```python
from build123d import *

# Parameters (mm, degrees)
F0_W      = 18.034
F0_H      = 23.4315
F1_DEPTH  = 21.0566
F2_W      = 18.034
F2_H      = 11.1252
F3_DEPTH  = 13.1699
F4_W      = 12.065
F4_H      = 4.5339
F5_DEPTH  = 12.065
F6_W      = 14.9352
F6_H      = 7.9248
F7_DEPTH  = 11.43
F8_W      = 11.3792
F8_H      = 3.8862
F9_DEPTH  = 11.43
F10_W     = 10.67195
F10_H     = 2.202249
F11_DEPTH = 11.176
F12_W     = 13.372126
F12_H     = 1.887192
F13_DEPTH = 10.922


with BuildPart() as f1:
    # F0 (on Front) → F1 (new body)
    with BuildSketch(Plane.XZ):
        Rectangle(F0_W, F0_H)
    extrude(amount=F1_DEPTH)

    # F2 (on face) → F3 (cut)
    with BuildSketch(Plane.XY.offset(11.71575)):
        with Locations((0, -15.494)):
            Rectangle(F2_W, F2_H)
    extrude(amount=-F3_DEPTH, mode=Mode.SUBTRACT)

    # F4 (on face) → F5 (join)
    with BuildSketch(Plane.XY.offset(11.71575)):
        with Locations((0, -4.9657)):
            Rectangle(F4_W, F4_H)
    extrude(amount=F5_DEPTH)

    # F6 (on face) → F7 (cut)
    with BuildSketch(Plane.XZ.offset(21.0566)):
        with Locations((0, -6.58495)):
            Rectangle(F6_W, F6_H)
    extrude(amount=-F7_DEPTH, mode=Mode.SUBTRACT)

    # F8 (on face) → F9 (cut)
    with BuildSketch(Plane.XY.offset(23.78075)):
        with Locations((0, -4.9657)):
            Rectangle(F8_W, F8_H)
    extrude(amount=-F9_DEPTH, mode=Mode.SUBTRACT)

    # F10 (on face) → F11 (join)
    with BuildSketch(Plane.XY.offset(12.35075)):
        with Locations((0, -4.296474)):
            Rectangle(F10_W, F10_H)
    extrude(amount=F11_DEPTH)

    # F12 (on face) → F13 (join)
    with BuildSketch(Plane.XZ.offset(9.6266)):
        with Locations((0, -5.182573)):
            Rectangle(F12_W, F12_H)
    extrude(amount=F13_DEPTH)


solid = f1.part
```
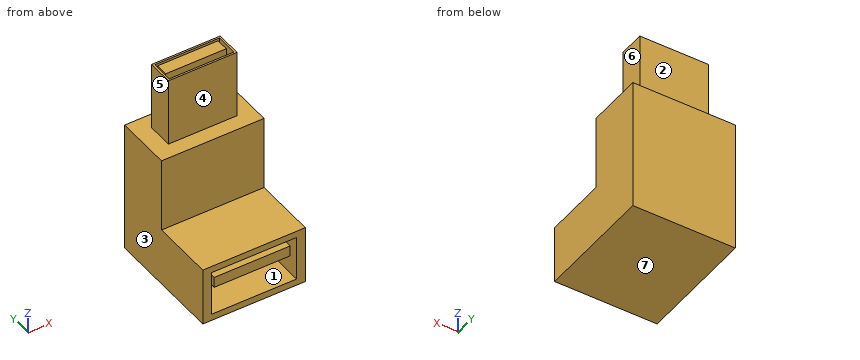
Part model, mm, in its own coordinate system. Face numbers are marked on the shaded views. A direction names the side the tool comes from. Round coordinates to 2 decimals unless told otherwise and drop trailing zeros. Loops run counter-clockwise (first coordinate to the right, second up) from the corner with the lowest first, then second, coordinate; pieces in that order, holes last. Notation, with made-up numbers: (82.5, -32) -> (136.5, -32) arc R14 cw to (136.5, -17) -> close; hole circle Ø2 at (-22, 19.5). An arc over 180 degrees is marked (long way). Use one line per item in the form item = value. Start each with the question number.
Item 1: Two-plate mould, pull along X, no slides. Class the marked faces 1, 2 and 3: released by +X, released by -X, zero draft, split by the parting line, or undercut.
Item 2: Band-saw the part on B-B (y = -10.5). List the corners of the cut face in (x, z), plus the area to 3 significant figures.
Item 3: Drop flat-ended pins along their axis: pin 1 Ø5 at (x, y) = (-4.5, -12.5) entering from +Z; pin 2 Ø5.5 at (x, z) = (-0.5, 18) entering from -Y; pin 3 Ø6 at (y, z) = (-5.5, 19) entering from +X. Give the stop position or say it passes through.
Item 4: Drill centre lines: line 1 along Y through (x, z) = (1.25, 18); line 2 along Z through (x, y) = (0.25, -15.25); line 3 along Z through (x, y) = (-7.25, -14.75). Where is each one in solid material? Low to high.
Item 5: Tool access for the marked faces 4, 5, 6 and 7: list every direction of +Z, -Z, +X, -X, +Y, -Y with a clear straight run to the whole face (end or side of a thin tool).
Item 6: Band-saw the part on D-D (y = -3.75). List the corners of the cut face in (x, z), plus the area to 3 significant figures.
Item 7: Band-saw the part on A-A (z = 15). List the corners of the cut face in (x, y).
Item 8: Band-saw the part on C-C (x = 1.25). List the corners of the cut face in (y, z), plus the area to 3 significant figures.
Data:
q1.face_1 = undercut
q1.face_2 = zero draft
q1.face_3 = released by -X
q2.outline = (-9.02, -11.72) -> (9.02, -11.72) -> (9.02, -1.45) -> (-9.02, -1.45) -> close; (-6.69, -6.13) -> (6.69, -6.13) -> (6.69, -4.24) -> (-6.69, -4.24) -> close; hole (-7.47, -10.55) -> (7.47, -10.55) -> (7.47, -2.62) -> (-7.47, -2.62) -> close
q2.area = 91.9 mm^2
q3.pin_1 = -1.45
q3.pin_2 = -7.23
q3.pin_3 = 6.03
q4.line_1 = -7.23 to -6.91, -5.4 to -3.2, -3.02 to -2.7
q4.line_2 = -11.72 to -10.55, -6.13 to -4.24, -2.62 to -1.45
q4.line_3 = -11.72 to -10.55, -2.62 to -1.45
q5.face_4 = +Z, +X, -X, -Y
q5.face_5 = +Z, -X, +Y, -Y
q5.face_6 = +Z, +X, +Y, -Y
q5.face_7 = -Z, +X, -X, +Y, -Y
q6.outline = (-9.02, -11.72) -> (9.02, -11.72) -> (9.02, 11.72) -> (6.03, 11.72) -> (6.03, 23.78) -> (5.69, 23.78) -> (5.69, 12.35) -> (5.34, 12.35) -> (5.34, 23.53) -> (-5.34, 23.53) -> (-5.34, 12.35) -> (-5.69, 12.35) -> (-5.69, 23.78) -> (-6.03, 23.78) -> (-6.03, 11.72) -> (-9.02, 11.72) -> close
q6.area = 557 mm^2
q7.outline = (-6.03, -7.23) -> (6.03, -7.23) -> (6.03, -2.7) -> (-6.03, -2.7) -> close; (-5.34, -5.4) -> (5.34, -5.4) -> (5.34, -3.2) -> (-5.34, -3.2) -> close; hole (-5.69, -6.91) -> (5.69, -6.91) -> (5.69, -3.02) -> (-5.69, -3.02) -> close
q8.outline = (-21.06, -11.72) -> (0, -11.72) -> (0, 11.72) -> (-2.7, 11.72) -> (-2.7, 23.78) -> (-3.02, 23.78) -> (-3.02, 12.35) -> (-3.2, 12.35) -> (-3.2, 23.53) -> (-5.4, 23.53) -> (-5.4, 12.35) -> (-6.91, 12.35) -> (-6.91, 23.78) -> (-7.23, 23.78) -> (-7.23, 11.72) -> (-9.93, 11.72) -> (-9.93, -1.45) -> (-21.06, -1.45) -> (-21.06, -2.62) -> (-9.63, -2.62) -> (-9.63, -4.24) -> (-20.55, -4.24) -> (-20.55, -6.13) -> (-9.63, -6.13) -> (-9.63, -10.55) -> (-21.06, -10.55) -> close
q8.area = 312 mm^2
